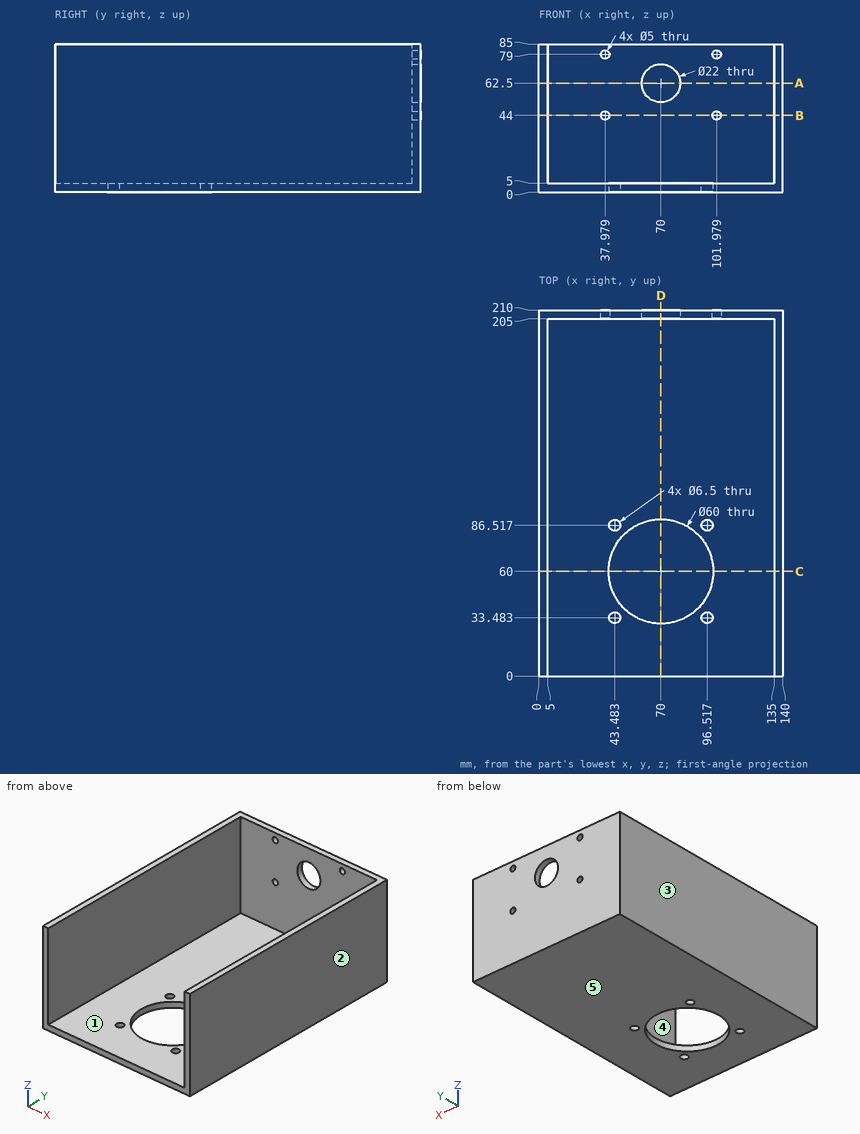
Check sheet for the drawn part. Datum: minimum x, y, z corner. Units: mm. A direction names the side the tool comes from. Give positions to 0.01 mm unless a question says otherwise; leave off trailing zeros. Order: outer loops, then holes, each group sorted by start corner. A loop starts at its lowest first (then second) coordinate and runs counter-clockwise, first axis right, second up. Notation, with made-up numbers: (59, 6.5) -> (89, 6.5) arc R26 cw to (89, 34.5) -> close; hole circle Ø2 at (11.25, 33.5). An arc over 180 degrees is marked (long way). Return JSON: item names as keys, results as strings.
1. Material ranges on probe 1 along X at (y, z) = (207.85, 44); probe 2 along X at (y, z) = (79, 29.5); probe 3 along Y at (x, z) = (70, 2), recorded low to high. Write a range as [from, to].
From the geometry:
{"probe 1": "[0, 35.48], [40.48, 99.48], [104.48, 140]", "probe 2": "[0, 5], [135, 140]", "probe 3": "[0, 30], [90, 210]"}
2. Cross-section at C-C, the plane y = 60. Record the cut outline in (x, z).
From the geometry:
{"outline": "(0, 0) -> (40, 0) -> (40, 5) -> (5, 5) -> (5, 85) -> (0, 85) -> close; (100, 0) -> (140, 0) -> (140, 85) -> (135, 85) -> (135, 5) -> (100, 5) -> close"}
3. Set-up check for the marked faces 1 and 2: record each of +Z, -Z, +X, -X, +Y, -Y from which the full face is reachable in a straight line by a thin tool's end or side.
From the geometry:
{"face 1": "+Z, -Y", "face 2": "+Z, -Z, +X, +Y, -Y"}
4. Cross-section at D-D, the plane x = 70. Record the cut outline in (y, z).
From the geometry:
{"outline": "(0, 0) -> (30, 0) -> (30, 5) -> (0, 5) -> close; (90, 0) -> (210, 0) -> (210, 51.5) -> (205, 51.5) -> (205, 5) -> (90, 5) -> close; (205, 73.5) -> (210, 73.5) -> (210, 85) -> (205, 85) -> close"}
5. Mould release check, pull along X, two halves, no side actions. Record for the marked faces 3, 4 and 5: +X half, -X half, draft (parallel to the pull), parting line (faces both ways), or undercut.
From the geometry:
{"face 3": "-X half", "face 4": "undercut", "face 5": "draft"}
6. Cross-section at A-A, the plane z = 62.5. Record the cut outline in (x, y), plus the area to 3 significant figures.
From the geometry:
{"outline": "(0, 0) -> (5, 0) -> (5, 205) -> (59, 205) -> (59, 210) -> (0, 210) -> close; (81, 205) -> (135, 205) -> (135, 0) -> (140, 0) -> (140, 210) -> (81, 210) -> close", "area": "2,640 mm^2"}
7. Go/stop test with flat-tipped pins: P1, Ø6.5, axis at x = 101.98, z = 79, coming from the +Y side; P2, Ø4, axis at x = 98, y = 48.5, coming from the +Z side; P3, Ø5, axis at x = 43.48, y = 86.52, coming from the -Z side; P4, Ø6, axis at x = 72, z = 45, coming from the -Y side. Record where each tip stops, or that it passes through.
From the geometry:
{"P1": "y = 210", "P2": "z = 5", "P3": "through", "P4": "y = 205"}
8. Cross-section at B-B, the plane z = 44. Record the cut outline in (x, y), plus the area to 3 significant figures.
From the geometry:
{"outline": "(0, 0) -> (5, 0) -> (5, 205) -> (35.48, 205) -> (35.48, 210) -> (0, 210) -> close; (40.48, 205) -> (99.48, 205) -> (99.48, 210) -> (40.48, 210) -> close; (104.48, 205) -> (135, 205) -> (135, 0) -> (140, 0) -> (140, 210) -> (104.48, 210) -> close", "area": "2,700 mm^2"}
